Check sheet for the modelled part. Datum: model origin and axes. Units: mm. Face numbers are marked on the shaded views. A direction names the side the tool comes from. Coordinates: 2 decimals unless noted, no trailing zeros. Order: outer loops, then holes, each group sorted by start corner. A loop starts at its lowest first (then second) coordinate and runs counter-clockwise, first axis right, second up.
1. Cross-section at C-C (x = 26.5). Enter the section's corners in (y, z).
2. Cross-section at A-A (z = 20). Enter the section's corners in (x, y), then the cut area to 3 significant figures.
3. Draft check along Z on the marked faces 3, 4, 5 and 6. Enter one of: released by +Z, released by -Z, zero draft, split by the parting line, or undercut.
4. Set-up check for the marked faces 1 and 2: record each of +Z, -Z, +X, -X, +Y, -Y from which the full face is reachable in a straight line by a thin tool's end or side.
5. Thickness scan on line 1 (X direction, y = 3.5, z = 20); line 2 (X direction, y = 8.25, z = -20); line 3 (X direction, y = 7.65, z = 20). Record the ranges inside material, lowest first.
6. Gauge pin test, flat ends, axial feed: pin 1 Ø7.5 at (x, z) = (26.5, -20) entering from +Y; pin 2 Ø1.3 at (x, y) = (-10, 7.5) entering from +Z. Record the tip position at first contact, or that the pin passes through.
7. Cross-section at D-D (y = 3). Enter the section's corners in (x, z).
8. Cross-section at B-B (y = 8.5). Enter the section's corners in (x, z), then the cut area to 3 significant figures.
```python
from build123d import *

# Parameters (mm, degrees)
SKETCH1_W                                           = 63
SKETCH1_H                                           = 50
BOSS_EXTRUDE1_DEPTH                                 = 9.3
CBORE_FOR_M5_HEX_SOCKET_HEAD_CAP_SCREW2_D           = 5.5
CBORE_FOR_M5_HEX_SOCKET_HEAD_CAP_SCREW2_CBORE_D     = 8.6
CBORE_FOR_M5_HEX_SOCKET_HEAD_CAP_SCREW2_CBORE_DEPTH = 4
CHAMFER1_SIZE                                       = 3
CHAMFER2_SIZE                                       = 2
CUT_EXTRUDE1_DEPTH                                  = 3
CUT_EXTRUDE2_DEPTH                                  = 4.3
SKETCH8_W                                           = 10
SKETCH8_H                                           = 19.9
CUT_EXTRUDE3_DEPTH                                  = 1.5


with BuildPart() as part:
    # Sketch1 → Boss-Extrude1 (new body)
    with BuildSketch(Plane(origin=(0, 0, 0), x_dir=(1, 0, 0), z_dir=(0, 1, 0))):
        Rectangle(SKETCH1_W, SKETCH1_H)
    extrude(amount=BOSS_EXTRUDE1_DEPTH)

    # CBORE for M5 Hex Socket Head Cap Screw2 (through all)
    with Locations(Plane(origin=(-26.5, 9.3, 20), x_dir=(0, 0, 1), z_dir=(0, 1, 0))):
        with Locations((0, 0), (0, 53), (-40, 53), (-40, 0)):
            CounterBoreHole(CBORE_FOR_M5_HEX_SOCKET_HEAD_CAP_SCREW2_D / 2, CBORE_FOR_M5_HEX_SOCKET_HEAD_CAP_SCREW2_CBORE_D / 2, CBORE_FOR_M5_HEX_SOCKET_HEAD_CAP_SCREW2_CBORE_DEPTH)

    # Chamfer1
    chamfer1_edges = [part.edges().sort_by_distance(p)[0] for p in [
        (-31.5, 4.65, -25),
        (31.5, 4.65, -25),
    ]]
    chamfer(chamfer1_edges, length=CHAMFER1_SIZE)

    # Chamfer2
    chamfer2_edges = [part.edges().sort_by_distance(p)[0] for p in [
        (31.5, 4.65, 25),
        (-31.5, 4.65, 25),
    ]]
    chamfer(chamfer2_edges, length=CHAMFER2_SIZE)

    # Sketch5 → Cut-Extrude1 (cut)
    with BuildSketch(Plane(origin=(0, 9.3, 0), x_dir=(1, 0, 0), z_dir=(0, 1, 0))):
        Polygon((0, -25), (-21.5, -25), (-21.5, 14.4), (21.5, 14.4), (21.5, -25), align=None)
    extrude(amount=-CUT_EXTRUDE1_DEPTH, mode=Mode.SUBTRACT)

    # Sketch7 → Cut-Extrude2 (cut)
    with BuildSketch(Plane(origin=(0, 9.3, 0), x_dir=(1, 0, 0), z_dir=(0, 1, 0))):
        Polygon((-21.5, 14.4), (31.5, 14.4), (31.5, 5), (-31.5, 5), (-31.5, 14.4), align=None)
    extrude(amount=-CUT_EXTRUDE2_DEPTH, mode=Mode.SUBTRACT)

    # Sketch8 → Cut-Extrude3 (cut)
    with BuildSketch(Plane(origin=(0, 9.3, 0), x_dir=(1, 0, 0), z_dir=(0, 1, 0))):
        with Locations((26.5, -4.95)):
            Rectangle(SKETCH8_W, SKETCH8_H)
        with Locations((-26.5, -4.95)):
            Rectangle(SKETCH8_W, SKETCH8_H)
    extrude(amount=-CUT_EXTRUDE3_DEPTH, mode=Mode.SUBTRACT)


solid = part.part
```
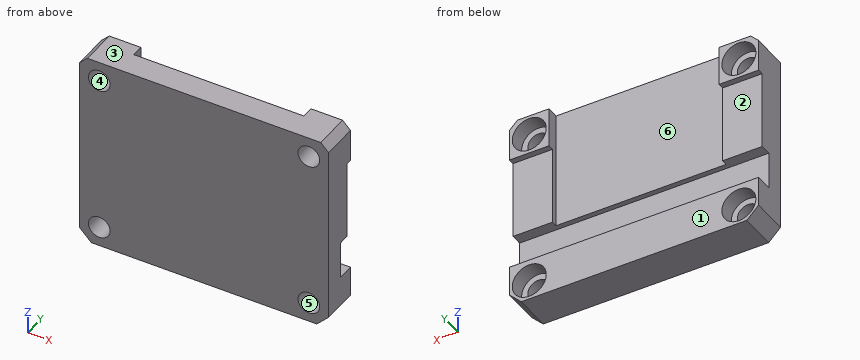
Data:
1. outline: (0, -25) - (9.3, -25) - (9.3, -24.3) - (5.3, -24.3) - (5.3, -22.75) - (0, -22.75) - close; (0, -17.25) - (5.3, -17.25) - (5.3, -15.7) - (9.3, -15.7) - (9.3, -14.4) - (5, -14.4) - (5, -5) - (7.8, -5) - (7.8, 14.9) - (9.3, 14.9) - (9.3, 15.7) - (5.3, 15.7) - (5.3, 17.25) - (0, 17.25) - close; (0, 22.75) - (5.3, 22.75) - (5.3, 24.3) - (9.3, 24.3) - (9.3, 25) - (0, 25) - close
2. outline: (-31.5, 0) - (-29.25, 0) - (-29.25, 5.3) - (-30.8, 5.3) - (-30.8, 9.3) - (-31.5, 9.3) - close; (-23.75, 0) - (23.75, 0) - (23.75, 5.3) - (22.2, 5.3) - (22.2, 9.3) - (21.5, 9.3) - (21.5, 6.3) - (-21.5, 6.3) - (-21.5, 9.3) - (-22.2, 9.3) - (-22.2, 5.3) - (-23.75, 5.3) - close; (29.25, 0) - (31.5, 0) - (31.5, 9.3) - (30.8, 9.3) - (30.8, 5.3) - (29.25, 5.3) - close
2. area: 330 mm2
3. face 3: released by +Z
3. face 4: undercut
3. face 5: undercut
3. face 6: zero draft
4. face 1: +Z, -Z, +X, -X, +Y
4. face 2: +X, -X, +Y
5. line 1: x = -31.5 to -29.25, -23.75 to 23.75, 29.25 to 31.5
5. line 2: x = -31.5 to -30.8, -22.2 to 22.2, 30.8 to 31.5
5. line 3: x = -31.5 to -30.8, -22.2 to -21.5, 21.5 to 22.2, 30.8 to 31.5
6. pin 1: stops at y = 5.3
6. pin 2: stops at z = -14.4
7. outline: (-31.5, -22) - (-28.5, -25) - (28.5, -25) - (31.5, -22) - (31.5, 23) - (29.5, 25) - (-29.5, 25) - (-31.5, 23) - close; hole circle Ø5.5 at (-26.5, -20); hole circle Ø5.5 at (-26.5, 20); hole circle Ø5.5 at (26.5, -20); hole circle Ø5.5 at (26.5, 20)
8. outline: (-31.5, -22) - (-28.5, -25) - (28.5, -25) - (31.5, -22) - (31.5, -14.4) - (-31.5, -14.4) - close; (-31.5, 14.9) - (-21.5, 14.9) - (-21.5, 25) - (-29.5, 25) - (-31.5, 23) - close; (21.5, 14.9) - (31.5, 14.9) - (31.5, 23) - (29.5, 25) - (21.5, 25) - close; hole circle Ø8.6 at (-26.5, -20); hole circle Ø8.6 at (-26.5, 20); hole circle Ø8.6 at (26.5, -20); hole circle Ø8.6 at (26.5, 20)
8. area: 624 mm2
